```python
from build123d import *

# Parameters (mm, degrees)
SKETCH_R        = 6
SKETCH_R_2      = 5
PAD_DEPTH       = 30
CHAMFER_SIZE    = 0.5
CHAMFER001_SIZE = 0.4
CHAMFER002_SIZE = 0.4


with BuildPart() as part:
    # Sketch → Pad (new body)
    with BuildSketch(Plane.XY):
        Circle(SKETCH_R)
        Circle(SKETCH_R_2, mode=Mode.SUBTRACT)
    extrude(amount=PAD_DEPTH)

    # Chamfer
    chamfer_edges = [part.edges().sort_by_distance(p)[0] for p in [
        (-6, 0, 30),
    ]]
    chamfer(chamfer_edges, length=CHAMFER_SIZE)

    # Chamfer001
    chamfer001_edges = [part.edges().sort_by_distance(p)[0] for p in [
        (-5, 0, 30),
    ]]
    chamfer(chamfer001_edges, length=CHAMFER001_SIZE)

    # Chamfer002
    chamfer002_edges = [part.edges().sort_by_distance(p)[0] for p in [
        (-5, 0, 0),
    ]]
    chamfer(chamfer002_edges, length=CHAMFER002_SIZE)


solid = part.part
```
The model under review builds one solid part; all positions refer to its coordinate system, in mm. Round coordinates to 2 decimals unless told otherwise and drop trailing zeros. Write each loop counter-clockwise with the first axis right and the second up, starting at its lowest first coordinate (ties: lowest second). Pieces come first, ordered by that corner, then holes. Notation, with made-up numbers: (67.25, 4) - (117.25, 4) arc R22 ccw to (117.25, 18) - close; hole circle Ø4 at (59, 74.25). An arc over 180 degrees is marked (long way). Use one line per item in the form item = value.
Q1. Consider section A-A (y = 0). State the section outline as (x, z) points.
Answer key:
outline = (-6, 0) - (-5.4, 0) - (-5, 0.4) - (-5, 29.6) - (-5.4, 30) - (-5.5, 30) - (-6, 29.5) - close; (5, 0.4) - (5.4, 0) - (6, 0) - (6, 29.5) - (5.5, 30) - (5.4, 30) - (5, 29.6) - close
Q2. Draft analysis for pull direction Y (two halves, no side actions). For faces 1 (the cylindrical face through (-6, 0, 15)), 2 (the cylindrical face through (-1.08, -4.88, 14.8)), state which applies: +Y half, -Y half, draft (parallel to the pull), parting line (faces both ways), or undercut.
Answer key:
face_1 = parting line
face_2 = undercut
Q3. For line 1 (Y direction, x = 0, z = 14.5); line 2 (Y direction, x = 3.25, z = 13.5); line 3 (X direction, y = -2.75, z = 4), list the stretches that pass through material, from the lowest coordinate up. Write a range as [from, to].
Answer key:
line_1 = [-6, -5], [5, 6]
line_2 = [-5.04, -3.8], [3.8, 5.04]
line_3 = [-5.33, -4.18], [4.18, 5.33]
Q4. Insertion check: pin 1 Ø2 at (y, z) = (-2, 27) entering from +X; pin 2 Ø4 at (x, y) = (-4, 0.5) entering from +Z; pin 3 Ø1 at (y, z) = (-2, 22.5) entering from -X; pin 4 Ø2 at (x, z) = (-2, 21.5) entering from +Y. Each pin has a flat end and moves straight along its axis. Give the tip position at first contact, or say it passes through.
Answer key:
pin_1 = 5.92
pin_2 = 30
pin_3 = -5.81
pin_4 = 5.92
